from build123d import *

# Parameters (mm, degrees)
F0_W     = 220
F0_H     = 330
F1_DEPTH = 60
F3_DEPTH = 60.001
F4_R     = 35
F5_DEPTH = 60.001


with BuildPart() as f1:
    # F0 (on Top) → F1 (new body)
    with BuildSketch(Plane.XY):
        Rectangle(F0_W, F0_H)
    extrude(amount=F1_DEPTH)

    # F2 (on face) → F3 (cut, through all)
    with BuildSketch(Plane.XY.offset(60)):
        with BuildLine():
            ThreePointArc((-28.722813, 110), (-31.024184, 146.201852), (0, 165))
            Line((0, 165), (-110, 165))
            Line((-110, 165), (-110, 110))
            Line((-110, 110), (-28.722813, 110))
        make_face()
        with BuildLine():
            ThreePointArc((0, 165), (31.024184, 146.201852), (28.722813, 110))
            Line((28.722813, 110), (110, 110))
            Line((110, 110), (110, 165))
            Line((110, 165), (0, 165))
        make_face()
        with BuildLine():
            Line((110, -165), (110, -110))
            Line((110, -110), (28.722813, -110))
            ThreePointArc((28.722813, -110), (31.024184, -146.201852), (0, -165))
            Line((0, -165), (110, -165))
        make_face()
        with BuildLine():
            Line((-110, -165), (0, -165))
            ThreePointArc((0, -165), (-31.024184, -146.201852), (-28.722813, -110))
            Line((-28.722813, -110), (-110, -110))
            Line((-110, -110), (-110, -165))
        make_face()
    extrude(amount=-F3_DEPTH, mode=Mode.SUBTRACT)

    # F4 (on face) → F5 (cut, through all)
    with BuildSketch(Plane.XY.offset(60)):
        with Locations((-90, 0)):
            Circle(F4_R)
        with Locations((90, 0)):
            Circle(F4_R)
    extrude(amount=-F5_DEPTH, mode=Mode.SUBTRACT)


solid = f1.part
The listing builds one solid part. Answer for the finished solid, in the listing's coordinates (mm). Coordinates: 2 decimals unless noted, no trailing zeros. Write each loop counter-clockwise with the first axis right and the second up, starting at its lowest first coordinate (ties: lowest second). Pieces come first, ordered by that corner, then holes. Notation, with made-up numbers: (73, 57) -> (104, 57) arc R22 ccw to (104, 72) -> close; hole circle Ø8 at (85, -32.75). An arc over 180 degrees is marked (long way). One line per question, with ' | ' between items.
1. Section C-C (y = 0) is taken. Determine the outline of the cut face in (x, z), and give its area (3 significant figures).
Verdict:
outline: (-55, 0) -> (55, 0) -> (55, 60) -> (-55, 60) -> close | area: 6,600 mm^2
2. Section D-D (x = 44) is taken. Determine the outline of the cut face in (y, z).
Verdict:
outline: (-110, 0) -> (110, 0) -> (110, 60) -> (-110, 60) -> close
3. Straight lines are drawn through the part: line 1 (Y direction, x = -90, z = 45.5); line 2 (Y direction, x = -88, z = 24); line 3 (Y direction, x = 53, z = 52). For each, find the intervals that lie inside material, in ascending order.
Verdict:
line 1: y = -110 to -35, 35 to 110 | line 2: y = -110 to -34.94, 34.94 to 110 | line 3: y = -110 to 110
4. Section A-A (x = -90) is taken. Determine the outline of the cut face in (y, z).
Verdict:
outline: (-110, 0) -> (-35, 0) -> (-35, 60) -> (-110, 60) -> close; (35, 0) -> (110, 0) -> (110, 60) -> (35, 60) -> close
5. Given pin 1 Ø12 at (y, z) = (-13, 48.5) entering from -X; pin 2 Ø3 at (x, z) = (26.5, 22) entering from -Y; pin 3 Ø6 at (y, z) = (-0.5, 32.5) entering from -X, each flat-ended and moving along its own axis, determine where each tip first touches the part or whether it passes through.
Verdict:
pin 1: stops at x = -60.61 | pin 2: stops at y = -154.49 | pin 3: stops at x = -55.18
6. For a pull along X with two mould halves and no side action, classify faces 1 (the flat face through (110, -70, 30)), 2 (the cylindrical face through (55.016, 1.068, 30.42)), 3 (the flat face through (-2, 2, 60)) as released by +X, released by -X, zero draft, split by the parting line, or undercut.
Verdict:
face 1: released by +X | face 2: undercut | face 3: zero draft
7. Section B-B (z = 43.5) is taken. Determine the outline of the cut face in (x, y), and give its area (3 significant figures).
Verdict:
outline: (-110, -110) -> (-28.72, -110) arc R35 ccw (long way) to (28.72, -110) -> (110, -110) -> (110, -28.72) arc R35 cw (long way) to (110, 28.72) -> (110, 110) -> (28.72, 110) arc R35 ccw (long way) to (-28.72, 110) -> (-110, 110) -> (-110, 28.72) arc R35 cw (long way) to (-110, -28.72) -> close | area: 48,400 mm^2
